Design review of the part built by this model. Coordinates are the model's own, in mm. A direction names the side the tool comes from. Coordinates: 2 decimals unless noted, no trailing zeros. Write each loop counter-clockwise with the first axis right and the second up, starting at its lowest first coordinate (ties: lowest second). Pieces come first, ordered by that corner, then holes. Notation, with made-up numbers: (42.5, -15.5) - (76.5, -15.5) arc R32 ccw to (76.5, 20.5) - close; hole circle Ø6 at (88.25, 9.5). An arc over 180 degrees is marked (long way). Answer as a JSON object with one key per item and string values.
```python
from build123d import *

# Parameters (mm, degrees)
SKETCH2_W           = 45
SKETCH2_H           = 23
BOSS_EXTRUDE1_DEPTH = 3
SKETCH3_W           = 15
SKETCH3_H           = 5
CUT_FOR_PINS_DEPTH  = 3
SKETCH6_W           = 15
SKETCH6_H           = 3
CUT_EXTRUDE3_DEPTH  = 3


with BuildPart() as part:
    # Sketch2 → Boss-Extrude1 (new body)
    with BuildSketch(Plane(origin=(0, 0, 0), x_dir=(1, 0, 0), z_dir=(0, 1, 0))):
        Rectangle(SKETCH2_W, SKETCH2_H)
    extrude(amount=BOSS_EXTRUDE1_DEPTH)

    # Sketch3 → cut for pins (cut)
    with BuildSketch(Plane(origin=(0, 3, 0), x_dir=(1, 0, 0), z_dir=(0, 1, 0))):
        with Locations((0, 9)):
            Rectangle(SKETCH3_W, SKETCH3_H)
    extrude(amount=-CUT_FOR_PINS_DEPTH, mode=Mode.SUBTRACT)

    # Sketch6 → Cut-Extrude3 (cut)
    with BuildSketch(Plane(origin=(0, 3, 0), x_dir=(1, 0, 0), z_dir=(0, 1, 0))):
        with Locations((-15, -10)):
            Rectangle(SKETCH6_W, SKETCH6_H)
        with Locations((15, -10)):
            Rectangle(SKETCH6_W, SKETCH6_H)
    extrude(amount=-CUT_EXTRUDE3_DEPTH, mode=Mode.SUBTRACT)


solid = part.part
```
(1) The part is to be moulded in two halves that separate along X. For faces 1 (the face through (-22.5, 1, -1)), 2 (the face through (0, 2, -6.5)), 3 (the face through (-15, 2, 8.5)), 4 (the face through (7.5, 2, -9)), say which applies: pulls with the +X half, pulls with the -X half, needs draft (parallel to the pull), parting line crosses it, or undercut.
Solved:
{"face 1": "pulls with the -X half", "face 2": "undercut", "face 3": "needs draft", "face 4": "undercut"}
(2) Take a section at A-A, the plane z = -8.5. Write out the cut boundary in (x, y), and give its area (3 significant figures).
Solved:
{"outline": "(-22.5, 0) - (-7.5, 0) - (-7.5, 3) - (-22.5, 3) - close; (7.5, 0) - (22.5, 0) - (22.5, 3) - (7.5, 3) - close", "area": "90.0 mm^2"}
(3) For pin 1 (8 mm diameter, centred on x = -8, z = 4.5, fed in from -Y), flat-tipped, find the tip position at first contact; note if it passes through.
Solved:
{"pin 1": "stops at y = 0"}
(4) To check wall thickness, follow line 1 (Z direction, x = -11, y = 2.8); line 2 (X direction, y = 2.7, z = -6.75); line 3 (Z direction, x = 3, y = 0.7). State the ranges of each line that lie inside material, in increasing order. Write a range as from..to.
Solved:
{"line 1": "z = -11.5..8.5", "line 2": "x = -22.5..-7.5, 7.5..22.5", "line 3": "z = -6.5..11.5"}
(5) Take a section at C-C, the plane x = 2. Write out the cut boundary in (y, z).
Solved:
{"outline": "(0, -6.5) - (3, -6.5) - (3, 11.5) - (0, 11.5) - close"}
(6) Take a section at B-B, the plane y = 0.6. Write out the cut boundary in (x, z), and give its area (3 significant figures).
Solved:
{"outline": "(-22.5, -11.5) - (-7.5, -11.5) - (-7.5, -6.5) - (7.5, -6.5) - (7.5, -11.5) - (22.5, -11.5) - (22.5, 8.5) - (7.5, 8.5) - (7.5, 11.5) - (-7.5, 11.5) - (-7.5, 8.5) - (-22.5, 8.5) - close", "area": "870 mm^2"}
(7) Take a section at D-D, the plane x = -18. Write out the cut boundary in (y, z), and give its area (3 significant figures).
Solved:
{"outline": "(0, -11.5) - (3, -11.5) - (3, 8.5) - (0, 8.5) - close", "area": "60.0 mm^2"}
(8) Tool access review of faces 5 (the face through (0, 0, 0)), 6 (the face through (-7.5, 2, 10)), 7 (the face through (-7.5, 2, -9)), 8 (the face through (7.5, 2, 10)), 9 (the face through (15, 1, -11.5)): name each direction out of +Z, -Z, +X, -X, +Y, -Y from which nothing blocks a thin tool from reaching the whole face with its end or side.
Solved:
{"face 5": "+Z, -Z, +X, -X, -Y", "face 6": "+Z, -X, +Y, -Y", "face 7": "-Z, +Y, -Y", "face 8": "+Z, +X, +Y, -Y", "face 9": "-Z, +X, -X, +Y, -Y"}
